Autodesk Fusion 360 part; units mm, degrees
sketch "Sketch1" plane through (0, 0, 0) normal (0, 1, 0) x (1, 0, 0)
  line L0 (0, -25) -> (23, -25)
  line L1 (25, -23) -> (25, 23)
  line L2 (23, 25) -> (0, 25)
  line L3 (0, -25) -> (-23, -25)
  line L4 (-25, -23) -> (-25, 23)
  line L5 (-23, 25) -> (0, 25)
  line L6 (0, -23) -> (-23, -23)
  line L7 (-23, -23) -> (-23, 23)
  line L8 (-23, 23) -> (0, 23)
  line L9 (23, 23) -> (0, 23)
  line L10 (23, -23) -> (23, 23)
  line L11 (0, -23) -> (23, -23)
  arc A0 (23, -25) -> (25, -23) centre (23, -23) ccw
  arc A1 (-25, -23) -> (-23, -25) centre (-23, -23) ccw
  arc A2 (-23, 25) -> (-25, 23) centre (-23, 23) ccw
  arc A3 (25, 23) -> (23, 25) centre (23, 23) ccw
  point P0 (25, -25)
  point P1 (25, 25)
  dimension "d1" = 25
  dimension "d2" = 25
  dimension "d3" = 50
  dimension "d4" = 2
  dimension "d7" = 2
  dimension "d8" = 2
  dimension "d9" = 2
  dimension "d10" = 2
extrude "Extrude1" add sketch "Sketch1" along normal blind 700
For this review, take the finished solid that the model builds, in its own axes (mm). A direction names the side the tool comes from. Give positions to 0.01 mm unless a question says otherwise; leave off trailing zeros. Write each loop counter-clockwise with the first axis right and the second up, starting at its lowest first coordinate (ties: lowest second). Pieces come first, ordered by that corner, then holes. Notation, with made-up numbers: M 85,43 L 126,43 A21 ccw 126,54 Z; hole C 29.5,-25 d2. An arc over 180 degrees is marked long. Answer as a JSON object with one key per item and string values. Group by question number.
Item 1: For probe 1 along X at (y, z) = (486.5, -16); probe 2 along X at (y, z) = (184, 23.5), list the stretches that pass through material, from the lowest coordinate up. Write a range as [from, to].
Item 2: Draft analysis for pull direction Z (two halves, no side actions). For faces 1 (the flat face through (0, 345, 25)), 2 (the flat face through (23, 345, 0)), 3 (the flat face through (-25, 345, 0)), state which applies: +Z half, -Z half, draft (parallel to the pull), parting line (faces both ways), or undercut.
Item 3: Consider section A-A on z = 5.5. Write out the cut boundary in (x, y).
Item 4: Consider section C-C on y = 614. Write out the cut boundary in (x, z).
Item 5: Consider section B-B on x = 0.5. Write out the cut boundary in (y, z).
Item 6: Tool access review of faces 4 (the flat face through (-2, 0, 24)), 5 (the flat face through (0, 345, 23)): name each direction out of +Z, -Z, +X, -X, +Y, -Y from which nothing blocks a thin tool from reaching the whole face with its end or side.
Check result:
{
 "1": {"probe 1": "x = [-25, -23], [23, 25]", "probe 2": "x = [-24.94, 24.94]"},
 "2": {"face 1": "+Z half", "face 2": "undercut", "face 3": "draft"},
 "3": {"outline": "M -25,0 L -23,0 L -23,700 L -25,700 Z; M 23,0 L 25,0 L 25,700 L 23,700 Z"},
 "4": {"outline": "M -25,-23 A2 ccw -23,-25 L 23,-25 A2 ccw 25,-23 L 25,23 A2 ccw 23,25 L -23,25 A2 ccw -25,23 Z; hole M -23,-23 L 23,-23 L 23,23 L -23,23 Z"},
 "5": {"outline": "M 0,-25 L 700,-25 L 700,-23 L 0,-23 Z; M 0,23 L 700,23 L 700,25 L 0,25 Z"},
 "6": {"face 4": "+Z, -Z, +X, -X, -Y", "face 5": "+Y, -Y"}
}
